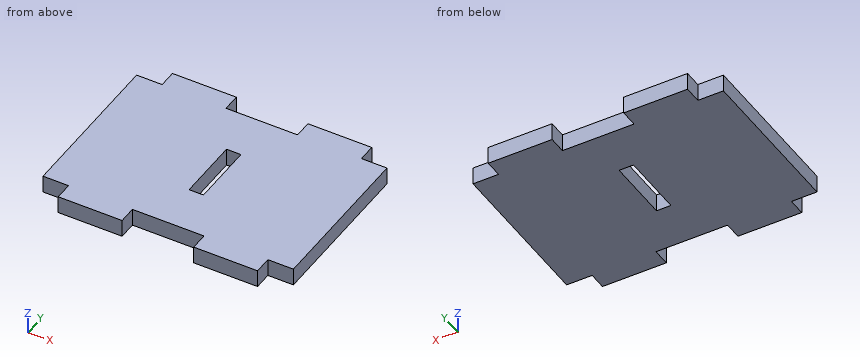
Autodesk Inventor part; units mm, degrees
ref_plane "YZ Plane" through (0, 0, 0) normal (1, 0, 0) x (0, 1, 0)
ref_plane "XZ Plane" through (0, 0, 0) normal (0, 1, 0) x (-1, 0, 0)
ref_plane "XY Plane" through (0, 0, 0) normal (0, 0, 1) x (1, 0, 0)
sketch "Sketch1" plane through (0, 0, 0) normal (0, 0, 1) x (1, 0, 0)
  line L0 (-12.089, 0) -> (-12.089, -5.5)
  line L1 (-12.089, -5.5) -> (-32.089, -5.5)
  line L2 (-32.089, -5.5) -> (-32.089, 0)
  line L3 (-54.514, 0) -> (-54.514, -5.5)
  line L4 (-54.514, -5.5) -> (-74.514, -5.5)
  line L5 (-74.514, -5.5) -> (-74.514, 0)
  line L6 (-32.089, 0) -> (-54.514, 0)
  line L7 (-12.089, 50) -> (-12.089, 55.5)
  line L8 (-12.089, 55.5) -> (-32.089, 55.5)
  line L9 (-32.089, 55.5) -> (-32.089, 50)
  line L10 (-54.514, 50) -> (-54.514, 55.5)
  line L11 (-54.514, 55.5) -> (-74.514, 55.5)
  line L12 (-74.514, 55.5) -> (-74.514, 50)
  line L13 (-32.089, 50) -> (-54.514, 50)
  line L14 (-12.089, 0) -> (-4.089, 0)
  line L15 (-4.089, 0) -> (-4.089, 50)
  line L16 (-4.089, 50) -> (-12.089, 50)
  line L17 (-74.514, 50) -> (-82.514, 50)
  line L18 (-82.514, 50) -> (-82.514, 0)
  line L19 (-82.514, 0) -> (-74.514, 0)
  dimension "d2" = 5.5
  dimension "d3" = 20
  dimension "d4" = 5.5
  dimension "d5" = 20
  dimension "d6" = 90
  dimension "d18" = 8
  dimension "d20" = 8
extrude "Extrusion1" add sketch "Sketch1" along normal blind 5.5
sketch "Sketch2" plane through (0, 0, 5.5) normal (0, 0, 1) x (1, 0, 0)
  line L0 (-43.3015, 15) -> (-45.5515, 15)
  line L1 (-45.5515, 15) -> (-45.5515, 35)
  line L2 (-45.5515, 35) -> (-43.3015, 35)
  line L3 (-43.3015, 15) -> (-41.0515, 15)
  line L4 (-41.0515, 15) -> (-41.0515, 35)
  line L5 (-41.0515, 35) -> (-43.3015, 35)
  point P0 (0, 0)
extrude "Extrusion2" cut sketch "Sketch2" against normal blind 10
properties part number "lado"
Design review of the part built by this model. Coordinates are the model's own, in mm. Round coordinates to 2 decimals unless told otherwise and drop trailing zeros. Order: outer loops, then holes, each group sorted by start corner. A loop starts at its lowest first (then second) coordinate and runs counter-clockwise, first axis right, second up.
1) Consider section A-A (z = 4.5). State the section outline as (x, y) points.
The answers:
outline: (-82.51, 0) - (-74.51, 0) - (-74.51, -5.5) - (-54.51, -5.5) - (-54.51, 0) - (-32.09, 0) - (-32.09, -5.5) - (-12.09, -5.5) - (-12.09, 0) - (-4.09, 0) - (-4.09, 50) - (-12.09, 50) - (-12.09, 55.5) - (-32.09, 55.5) - (-32.09, 50) - (-54.51, 50) - (-54.51, 55.5) - (-74.51, 55.5) - (-74.51, 50) - (-82.51, 50) - close; hole (-45.55, 15) - (-41.05, 15) - (-41.05, 35) - (-45.55, 35) - close
2) Consider section B-B (y = 20). State the section outline as (x, z) points, plus the area to 3 significant figures.
The answers:
outline: (-82.51, 0) - (-45.55, 0) - (-45.55, 5.5) - (-82.51, 5.5) - close; (-41.05, 0) - (-4.09, 0) - (-4.09, 5.5) - (-41.05, 5.5) - close
area: 407 mm2
3) Clearance check with flat-ended pins moving along their axes: pin 1 Ø3 at (y, z) = (-3.5, 2) entering from +X; pin 2 Ø1.6 at (x, z) = (-44, 2) entering from +Y; pin 3 Ø1.6 at (y, z) = (51.5, 3.5) entering from -X; pin 4 Ø10 at (x, y) = (-70, 27) entering from -Z. State where each tip first meets the part, or that it passes through.
The answers:
pin 1: stops at x = -12.09
pin 2: stops at y = 50
pin 3: stops at x = -74.51
pin 4: stops at z = 0
4) For L1, parallel to X at y = 21.5, z = 1.65; L2, parallel to Y at x = -44, z = 3.75; L3, parallel to Y at x = -77, z = 3.6, list the stretches that pass through material, from the lowest coordinate up.
The answers:
L1: x = -82.51 to -45.55, -41.05 to -4.09
L2: y = 0 to 15, 35 to 50
L3: y = 0 to 50
5) Consider section C-C (x = -40). State the section outline as (y, z) points, plus the area to 3 significant figures.
The answers:
outline: (0, 0) - (50, 0) - (50, 5.5) - (0, 5.5) - close
area: 275 mm2
